Autodesk Fusion 360 part; units mm, degrees
sketch "Sketch1" plane through (0, 0, 0) normal (1, 0, 0) x (0, 1, 0)
  line L0 (77.85, 0) -> (77.85, 20)
  line L1 (0, 10) -> (-14.9603, 10) construction
  line L2 (-4.15, 16) -> (0, 14.4895)
  line L3 (-7.2644, 13.9) -> (-10.25, 13.1)
  line L4 (0, 6.9) -> (-6, 6.9)
  line L5 (0, 20) -> (-4.15, 20)
  line L6 (0, 0) -> (77.85, 0)
  line L7 (-10.25, 6.9) -> (-10.25, 8.1)
  line L8 (-6, 6.9) -> (-7.2644, 6.1)
  line L9 (-10.25, 8.1) -> (0, 8.1)
  line L10 (-4.15, 4) -> (0, 5.5105)
  line L11 (-10.25, 13.1) -> (-10.25, 11.9)
  line L12 (-7.2644, 6.1) -> (-10.25, 6.9)
  line L13 (0, 10) -> (-14.9603, 10) construction
  line L14 (-4.15, 20) -> (-4.15, 16)
  line L15 (-4.15, 0) -> (-4.15, 4)
  line L16 (0, 20) -> (0, 0)
  line L17 (-6, 13.1) -> (-7.2644, 13.9)
  line L18 (0, 0) -> (-4.15, 0)
  line L19 (77.85, 0) -> (77.85, 20)
  line L20 (-10.25, 11.9) -> (0, 11.9)
  line L21 (0, 13.1) -> (-6, 13.1)
  line L22 (77.85, 20) -> (0, 20)
  dimension "d1" = 20
  dimension "d2" = 6
  dimension "d3" = 1.85
  dimension "d4" = 4
  dimension "d5" = 1.2
  dimension "d6" = 4.25
  dimension "d7" = 3.1
  dimension "d8" = 70
  dimension "d9" = 0.8
  dimension "d10" = 105
  dimension "d14" = 20
  dimension "d21" = 82
extrude "Extrude1" add sketch "Sketch1" along normal blind 20
Geometry: final body of the model. Coordinates: model frame, mm. A direction names the side the tool comes from. Coordinates: 2 decimals unless noted, no trailing zeros. Order: outer loops, then holes, each group sorted by start corner. A loop starts at its lowest first (then second) coordinate and runs counter-clockwise, first axis right, second up. Notation, with made-up numbers: M -19,53.25 L 22,53.25 A20 cw 22,77.25 Z; hole C 12.5,41.25 d3. An arc over 180 degrees is marked long. Answer in a Markdown table with one row per item. Add a question column.
Q1. Mould query, pull axis Z, two halves, no side actions, for faces 5 (the flat face through (9.86, -2.104, 4.745)), 6 (the flat face through (0, 33, 10)), 7 (the flat face through (9.86, -8.736, 13.506)), 8 (the flat face through (9.86, -8.736, 6.494)). Classes: released by +Z, released by -Z, zero draft, split by the parting line, or undercut.
Q2. Section query A-A on x = 10. Return the cut outline in (y, z).
Q3. Section query C-C on z = 10.25. Return the cut outline in (x, y).
Q4. Contact query for flat-ended pins moving along their axis: P1, Ø3, axis at x = 11.5, z = 2, coming from the -Y side; P2, Ø1.5, axis at x = 10, z = 11, coming from the -Y side. Output: stop coordinate, or through.
Q5. Line query: L1, parallel to Y at x = 16.75, z = 3.25; L2, parallel to Z at x = 12.25, y = -6; L3, parallel to Y at x = 13.5, z = 6. Output: solid intervals per line, ascending.
Q6. Section query B-B on y = -2. Return the cut outline in (x, z).
Q7. Reachability of faces 1 (the flat face through (10, -4.15, 2)), 2 (the flat face through (10, -4.15, 18)), 3 (the flat face through (10, 0, 10)), 4 (the flat face through (10, 0, 6)) from +Z, -Z, +X, -X, +Y, -Y: full face, straight path, thin tool, end or side. Return the list, or none.
Q8. Section query D-D on z = 3. Return the cut outline in (x, y), and give its area (3 significant figures).
Completed:
| question | item | result |
|---|---|---|
| 1 | face 5 | undercut |
| 1 | face 6 | zero draft |
| 1 | face 7 | released by +Z |
| 1 | face 8 | released by -Z |
| 2 | outline | M -10.25,6.9 L -7.26,6.1 L -6,6.9 L 0,6.9 L 0,5.51 L -4.15,4 L -4.15,0 L 77.85,0 L 77.85,20 L -4.15,20 L -4.15,16 L 0,14.49 L 0,13.1 L -6,13.1 L -7.26,13.9 L -10.25,13.1 L -10.25,11.9 L 0,11.9 L 0,8.1 L -10.25,8.1 Z |
| 3 | outline | M 0,0 L 20,0 L 20,77.85 L 0,77.85 Z |
| 4 | P1 | stops at y = -4.15 |
| 4 | P2 | stops at y = 0 |
| 5 | L1 | y = -4.15 to 77.85 |
| 5 | L2 | z = 6.9 to 8.1, 11.9 to 13.1 |
| 5 | L3 | y = 0 to 77.85 |
| 6 | outline | M 0,0 L 20,0 L 20,4.78 L 0,4.78 Z; M 0,6.9 L 20,6.9 L 20,8.1 L 0,8.1 Z; M 0,11.9 L 20,11.9 L 20,13.1 L 0,13.1 Z; M 0,15.22 L 20,15.22 L 20,20 L 0,20 Z |
| 7 | face 1 | -Z, +X, -X, -Y |
| 7 | face 2 | +Z, +X, -X, -Y |
| 7 | face 3 | +X, -X, -Y |
| 7 | face 4 | +X, -X |
| 8 | outline | M 0,-4.15 L 20,-4.15 L 20,77.85 L 0,77.85 Z |
| 8 | area | 1,640 mm2 |
